from build123d import *

# Parameters (mm, degrees)
SKETCH1_R           = 4
SKETCH1_W           = 15
SKETCH1_H           = 15
BOSS_EXTRUDE1_DEPTH = 15


with BuildPart() as part:
    # Sketch1 → Boss-Extrude1 (new body)
    with BuildSketch(Plane.XY):
        Polygon((0, 0), (0, 80), (444, 80), (444, 0), (336.25, 0), (336.25, 15), (316.25, 15), (316.25, 0), (232.5, 0), (232.5, 15), (212.5, 15), (212.5, 0), (128.75, 0), (128.75, 15), (108.75, 15), (108.75, 0), align=None)
        with Locations((44, 66)):
            Circle(SKETCH1_R, mode=Mode.SUBTRACT)
        with Locations(Location((400, 66, 0), (0, 0, 180))):  # turned: the seam where the file's is
            Circle(SKETCH1_R, mode=Mode.SUBTRACT)
        with Locations((17.5, 60)):
            Rectangle(SKETCH1_W, SKETCH1_H, mode=Mode.SUBTRACT)
        with Locations((17.5, 20)):
            Rectangle(SKETCH1_W, SKETCH1_H, mode=Mode.SUBTRACT)
        with Locations((426.5, 20)):
            Rectangle(SKETCH1_W, SKETCH1_H, mode=Mode.SUBTRACT)
        with Locations((426.5, 60)):
            Rectangle(SKETCH1_W, SKETCH1_H, mode=Mode.SUBTRACT)
    extrude(amount=BOSS_EXTRUDE1_DEPTH)


solid = part.part
Part model, mm, in its own coordinate system. A direction names the side the tool comes from. Coordinates: 2 decimals unless noted, no trailing zeros. Loops run counter-clockwise (first coordinate to the right, second up) from the corner with the lowest first, then second, coordinate; pieces in that order, holes last. Notation, with made-up numbers: (22, 54.25) - (67, 54.25) arc R26 ccw to (67, 88.25) - close; hole circle Ø10 at (-12, 0.5). An arc over 180 degrees is marked (long way). Write each question's results on one line, items separated by ' | '. Start each with the question number.
Q1. Drop a flat-ended pin along its axis: pin 1 Ø6.5 at (x, y) = (400, 66) entering from +Z (1 decimal). Give the stop position or say it passes through.
Q2. Two-plate mould, pull along Y, no slides. Class faces 4 (the flat face through (128.75, 7, 7)), 5 (the flat face through (17, 52.5, 7)), 6 (the flat face through (275, 0, 7)): +Y half, -Y half, draft (parallel to the pull), parting line (faces both ways), or undercut.
Q3. Slice it at C-C on z = 3. Give the number of separate pieces and of enclosed holes in the cut face, and give its area (3 significant figures).
Q4. Slice it at A-A on y = 20.5. Give the cut face in (x, z), and give its area (3 significant figures).
Q5. Which spindle directions (+Z, -Z, +X, -X, +Y, -Y) get a long thin tool onto all of the face, cutting with end or side? Do faces 1 (the flat face through (212.5, 8, 7)), 2 (the flat face through (219, 80, 7)), 3 (the flat face through (25, 20, 7)). Say none if no direction does.
Q6. Slice it at B-B on x = 44. Give the cut face in (y, z), and give its area (3 significant figures).
Q7. Probe line 1 along X through (y, z) = (19.5, 9); line 2 along Y through (x, z) = (400, 7.5); line 3 along X through (y, z) = (63, 8). List the from-to ranges inside material, lowest first.
Answer:
1) pin 1: passes through
2) face 4: draft | face 5: undercut | face 6: -Y half
3) separate pieces: 1 | enclosed holes: 6 | area: 33,600 mm2
4) outline: (0, 0) - (10, 0) - (10, 15) - (0, 15) - close; (25, 0) - (419, 0) - (419, 15) - (25, 15) - close; (434, 0) - (444, 0) - (444, 15) - (434, 15) - close | area: 6,210 mm2
5) face 1: +Z, -Z, -Y | face 2: +Z, -Z, +X, -X, +Y | face 3: +Z, -Z
6) outline: (0, 0) - (62, 0) - (62, 15) - (0, 15) - close; (70, 0) - (80, 0) - (80, 15) - (70, 15) - close | area: 1,080 mm2
7) line 1: x = 0 to 10, 25 to 419, 434 to 444 | line 2: y = 0 to 62, 70 to 80 | line 3: x = 0 to 10, 25 to 41.35, 46.65 to 397.35, 402.65 to 419, 434 to 444
